```python
from build123d import *

# Parameters (mm, degrees)
SKETCH_2_R          = 19
SKETCH_2_R_2        = 2.75
EXTRUDE_1_DEPTH     = 13.9
SKETCH_3_R          = 21.125
CUT_EXTRUDE_1_DEPTH = 12.15
SKETCH_4_R          = 5
CUT_EXTRUDE_2_DEPTH = 8.9
FILLET_1_R          = 8
EXTRUDE_START       = 2
SKETCH_7_R          = 0.9
EXTRUDE_2_DEPTH     = 2
SKETCH_5_R          = 0.9
CUT_EXTRUDE_3_DEPTH = 61.488614631
FILLET_2_R          = 8


with BuildPart() as part:
    # Эскиз2 → Бобышка-Вытянуть1 (new body)
    with BuildSketch(Plane.XY):
        with BuildLine():
            ThreePointArc((26, 26.25), (0, 52.25), (-26, 26.25))
            Line((-26, 26.25), (-26, -20))
            Line((-26, -20), (26, -20))
            Line((26, -20), (26, 26.25))
        make_face()
        with Locations((0, 26.25)):
            Circle(SKETCH_2_R, mode=Mode.SUBTRACT)
        with Locations((12, -10)):
            Circle(SKETCH_2_R_2, mode=Mode.SUBTRACT)
        with Locations((-12, -10)):
            Circle(SKETCH_2_R_2, mode=Mode.SUBTRACT)
    extrude(amount=EXTRUDE_1_DEPTH)

    # Эскиз3 → Вырез-Вытянуть1 (cut)
    with BuildSketch(Plane.XY.offset(13.9)):
        with Locations((0, 26.25)):
            Circle(SKETCH_3_R)
    extrude(amount=-CUT_EXTRUDE_1_DEPTH, mode=Mode.SUBTRACT)

    # Эскиз4 → Вырез-Вытянуть2 (cut)
    with BuildSketch(Plane(origin=(0, 0, 0), x_dir=(-1, 0, 0), z_dir=(0, 0, -1))):
        with Locations((-12, -10)):
            Circle(SKETCH_4_R)
        with Locations((12, -10)):
            Circle(SKETCH_4_R)
    extrude(amount=-CUT_EXTRUDE_2_DEPTH, mode=Mode.SUBTRACT)

    # Скругление1
    fillet_1_edges = [part.edges().sort_by_distance(p)[0] for p in [
        (26, -20, 6.95),
        (-26, -20, 6.95),
    ]]
    fillet(fillet_1_edges, radius=FILLET_1_R)

    # Эскиз7 → Бобышка-Вытянуть2 (add)
    # profile 1 of 2: a face of its own
    with BuildSketch(Plane(origin=(0, 0, 0), x_dir=(-1, 0, 0), z_dir=(0, 0, -1)).offset(EXTRUDE_START)):
        with BuildLine():
            Line((-24.571324751, 34.75), (-9.2, 34.75))
            ThreePointArc((-9.2, 34.75), (-7.078679656, 33.871320344), (-6.2, 31.75))
            Line((-6.2, 31.75), (-6.2, 20.75))
            ThreePointArc((-6.2, 20.75), (-7.078679656, 18.628679656), (-9.2, 17.75))
            Line((-9.2, 17.75), (-26, 17.75))
            Line((-26, 17.75), (-26, 26.25))
            ThreePointArc((-26, 26.25), (-25.640343636, 30.559614628), (-24.571324751, 34.75))
        make_face()
        with Locations((-9.2, 31.75)):
            Circle(SKETCH_7_R, mode=Mode.SUBTRACT)
        with Locations((-9.2, 20.75)):
            Circle(SKETCH_7_R, mode=Mode.SUBTRACT)
    # profile 2 of 2: a face of its own
    with BuildSketch(Plane(origin=(0, 0, 0), x_dir=(-1, 0, 0), z_dir=(0, 0, -1)).offset(EXTRUDE_START)):
        with BuildLine():
            Line((26, 26.25), (26, 17.75))
            Line((26, 17.75), (9.2, 17.75))
            ThreePointArc((9.2, 17.75), (7.078679656, 18.628679656), (6.2, 20.75))
            Line((6.2, 20.75), (6.2, 31.75))
            ThreePointArc((6.2, 31.75), (7.078679656, 33.871320344), (9.2, 34.75))
            Line((9.2, 34.75), (24.571324751, 34.75))
            ThreePointArc((24.571324751, 34.75), (25.640343636, 30.559614628), (26, 26.25))
        make_face()
        with Locations(Location((9.2, 20.75, 0), (0, 0, 180))):
            Circle(SKETCH_7_R, mode=Mode.SUBTRACT)
        with Locations(Location((9.2, 31.75, 0), (0, 0, 180))):
            Circle(SKETCH_7_R, mode=Mode.SUBTRACT)
    extrude(amount=-EXTRUDE_2_DEPTH)

    # Эскиз5 → Вырез-Вытянуть3 (cut, through all)
    with BuildSketch(Plane.XY.offset(13.9)):
        with Locations((0, 49.75)):
            Circle(SKETCH_5_R)
        with Locations((-23.5, 26.25)):
            Circle(SKETCH_5_R)
        with Locations((0, 2.75)):
            Circle(SKETCH_5_R)
        with Locations((23.5, 26.25)):
            Circle(SKETCH_5_R)
        with Locations((-22, -10)):
            Circle(SKETCH_5_R)
        with Locations((22, -10)):
            Circle(SKETCH_5_R)
    extrude(amount=-CUT_EXTRUDE_3_DEPTH, mode=Mode.SUBTRACT)

    # Скругление2
    # the kernel refuses this fillet: 8 mm, written as the material it adds along each edge
    with BuildSketch(Plane(origin=(0, 26.25, 0), x_dir=(1, 0, 0), z_dir=(0, -1, 0))) as fillet_2_piece_1_section:
        with BuildLine():
            CenterArc((14.006253911, 8), FILLET_2_R, 270, 38.624832873)
            Line((14.006253911, 0), (19, 0))
            Line((19, 0), (19, 1.75))
        make_face()
    fillet_2_piece_1 = revolve(axis=Axis((0, 26.25, 0), (0, 0, 1)), revolution_arc=64.223731821, mode=Mode.PRIVATE)
    fillet_2_piece_1 = split(fillet_2_piece_1, bisect_by=Plane(origin=(15.779655811, 34.75, 0.435065896), z_dir=(0, -1, 0)), keep=Keep.TOP, mode=Mode.PRIVATE)
    add(fillet_2_piece_1)
    with BuildSketch(Plane(origin=(0, 26.25, 0), x_dir=(-0.43479598917537754, 0.900528982208238, 0), z_dir=(0.900528982208238, 0.43479598917537754, 0))) as fillet_2_piece_2_section:
        with BuildLine():
            CenterArc((14.006253911, 8), FILLET_2_R, 270, 38.624832873)
            Line((14.006253911, 0), (19, 0))
            Line((19, 0), (19, 1.75))
        make_face()
    fillet_2_piece_2 = revolve(axis=Axis((0, 26.25, 0), (0, 0, 1)), revolution_arc=128.45537387, mode=Mode.PRIVATE)
    fillet_2_piece_2 = split(fillet_2_piece_2, bisect_by=Plane(origin=(-16.657296725, 17.75, 0.435065896), z_dir=(0, 1, 0)), keep=Keep.TOP, mode=Mode.PRIVATE)
    fillet_2_piece_2 = split(fillet_2_piece_2, bisect_by=Plane(origin=(-16.657296725, 34.75, 0.435065896), z_dir=(0, -1, 0)), keep=Keep.TOP, mode=Mode.PRIVATE)
    add(fillet_2_piece_2)
    with BuildSketch(Plane(origin=(0, 26.25, 0), x_dir=(0.43485815144729206, -0.9004989661958774, 0), z_dir=(-0.9004989661958774, -0.43485815144729206, 0))) as fillet_2_piece_3_section:
        with BuildLine():
            CenterArc((14.006253911, 8), FILLET_2_R, 270, 38.624832873)
            Line((14.006253911, 0), (19, 0))
            Line((19, 0), (19, 1.75))
        make_face()
    fillet_2_piece_3 = revolve(axis=Axis((0, 26.25, 0), (0, 0, 1)), revolution_arc=64.223731821, mode=Mode.PRIVATE)
    fillet_2_piece_3 = split(fillet_2_piece_3, bisect_by=Plane(origin=(15.779655811, 17.75, 0.435065896), z_dir=(0, 1, 0)), keep=Keep.TOP, mode=Mode.PRIVATE)
    add(fillet_2_piece_3)


solid = part.part
```
Could you check a few things on this model? Use its own coordinates, in mm. A direction names the side the tool comes from. Coordinates: 2 decimals unless noted, no trailing zeros. Order: outer loops, then holes, each group sorted by start corner. A loop starts at its lowest first (then second) coordinate and runs counter-clockwise, first axis right, second up. Notation, with made-up numbers: M 17,28.25 L 65,28.25 A24 cw 65,58.25 Z; hole C 86.25,-33.75 d9. An arc over 180 degrees is marked long. Use one line per item in the form item = value. Start each with the question number.
1. For pin 1 (21 mm diameter, centred on x = 6.5, y = 27.5, fed in from +Z); pin 2 (0.6 mm diameter, centred on y = 28.5, z = -1, fed in from +X); pin 3 (3 mm diameter, centred on x = 22, y = -10, fed in from -Z); pin 4 (1.4 mm diameter, centred on x = -9.2, y = 20.75, fed in from -Z), each with a flat end and sliding along its axis, tell me the tip position at first contact or that it passes through.
2. We'd pull the mould along Y, two halves only. Please class faces 1 (the cylindrical face through (-24, 27, 6)), 2 (the flat face through (-6.2, 26, -1)), 3 (the cylindrical face through (23.719, -17.594, 7.047)): +Y half, -Y half, draft (parallel to the pull), parting line (faces both ways), or undercut.
3. Please list where these lines run through material, in increasing order: line 1 (Y direction, x = 0, z = 8.25) (3 decimals); line 2 (Y direction, x = 13.5, z = 0.5); line 3 (Y direction, x = -13, z = 2.25).
4. Suppose I cut it at A-A on y = 2.75. Write out the boundary of the cut face in (x, z), then the cut area to 3 significant figures.
5. On a 3-axis mill with a long thin cutter (end or side, diameter ignored), from which of +Z, -Z, +X, -X, +Y, -Y can I reach the whole of each face in a straight line? I mean faces 4 (the flat face through (6.2, 26, -1)), 5 (the flat face through (-19, 29, 1.75)), 6 (the cylindrical face through (-7.06, 33.85, -1.01)). Say none if no direction works.
6. Suppose I cut it at D-D on y = 49.75. Write out the boundary of the cut face in (x, z).
7. Suppose I cut it at B-B on z = 7.25. Count the separate pieces of the cut face and the enclosed holes in it, then the cut area to 3 significant figures.
Geometry says:
q1.pin_1 = 0.63
q1.pin_2 = 25.93
q1.pin_3 = 0
q1.pin_4 = through
q2.face_1 = undercut
q2.face_2 = draft
q2.face_3 = -Y half
q3.line_1 = -20 to 1.85, 3.65 to 5.125, 47.375 to 48.85, 50.65 to 52.25
q3.line_2 = -20 to -14.77, -5.23 to 12.88, 39.62 to 48.47
q3.line_3 = -20 to -14.9, -5.1 to 9.6, 42.9 to 48.77
q4.outline = M -26,0 L -0.9,0 L -0.9,13.9 L -26,13.9 Z; M 0.9,0 L 26,0 L 26,13.9 L 0.9,13.9 Z
q4.area = 698 mm^2
q5.face_4 = +Z, -Z, +Y, -Y
q5.face_5 = +Z
q5.face_6 = +Z, -Z, +Y
q6.outline = M -11.12,0 L -0.9,0 L -0.9,13.9 L -11.12,13.9 Z; M 0.9,0 L 11.12,0 L 11.12,13.9 L 0.9,13.9 Z
q7.separate_pieces = 1
q7.enclosed_holes = 9
q7.area = 1,870 mm^2
